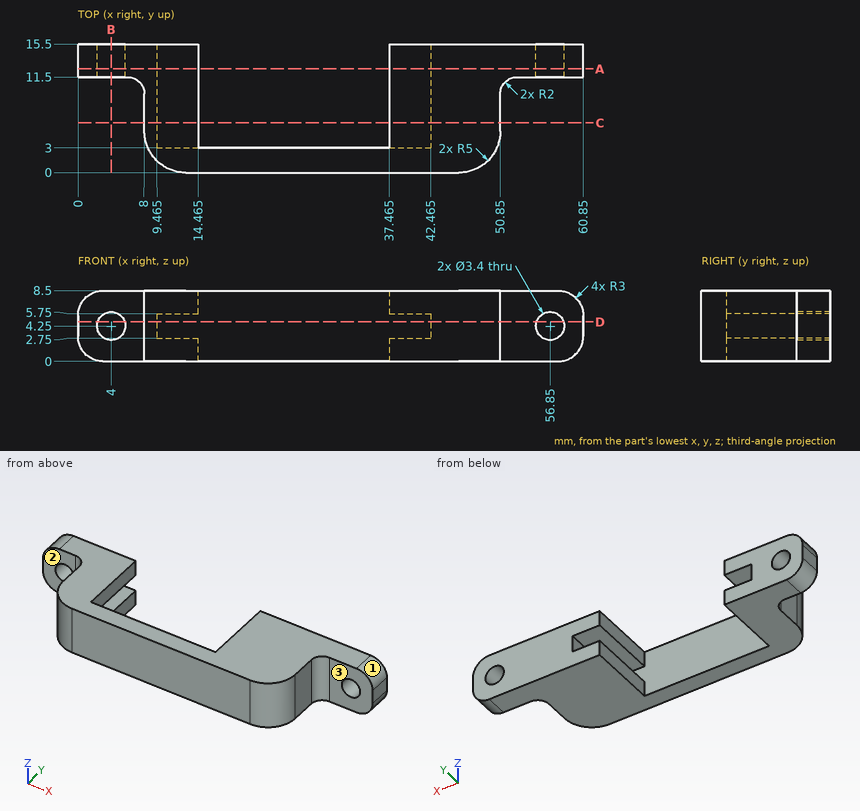
Part print with two shaded views. Sizes in mm from the minimum x, y, z corner. A direction names the side the tool comes from. Round coordinates to 2 decimals unless told otherwise and drop trailing zeros. Write each loop counter-clockwise with the first axis right and the second up, starting at its lowest first coordinate (ties: lowest second). Pieces come first, ordered by that corner, then holes. Notation, with made-up numbers: (41, -4) - (60, -4) arc R24 ccw to (60, 10) - close; hole circle Ø9 at (42.25, 81.5). An arc over 180 degrees is marked (long way). Use CSV: the item, a comma, the result in double quotes.
Item 1: Slice it at A-A, the plane y = 12.5. Write the cut outline in (x, z) (3 decimals), then the cut area to 3 significant figures.
Results list:
outline,"(0, 3) arc R3 ccw to (3, 0) - (14.465, 0) - (14.465, 2.75) - (9.465, 2.75) - (9.465, 5.75) - (14.465, 5.75) - (14.465, 8.5) - (3, 8.5) arc R3 ccw to (0, 5.5) - close; (37.465, 0) - (57.85, 0) arc R3 ccw to (60.85, 3) - (60.85, 5.5) arc R3 ccw to (57.85, 8.5) - (37.465, 8.5) - (37.465, 5.75) - (42.465, 5.75) - (42.465, 2.75) - (37.465, 2.75) - close; hole circle Ø3.4 at (4, 4.25); hole circle Ø3.4 at (56.85, 4.25)"
area,"266 mm²"
Item 2: Slice it at B-B, the plane x = 4. Write the cut outline in (y, z), then the cut area to 3 significant figures.
Results list:
outline,"(11.5, 0) - (15.5, 0) - (15.5, 2.55) - (11.5, 2.55) - close; (11.5, 5.95) - (15.5, 5.95) - (15.5, 8.5) - (11.5, 8.5) - close"
area,"20.4 mm²"
Item 3: Slice it at C-C, the plane y = 6. Write the cut outline in (x, z) (3 decimals), then the cut area to 3 significant figures.
Results list:
outline,"(8, 0) - (14.465, 0) - (14.465, 2.75) - (9.465, 2.75) - (9.465, 5.75) - (14.465, 5.75) - (14.465, 8.5) - (8, 8.5) - close; (37.465, 0) - (50.85, 0) - (50.85, 8.5) - (37.465, 8.5) - (37.465, 5.75) - (42.465, 5.75) - (42.465, 2.75) - (37.465, 2.75) - close"
area,"139 mm²"
Item 4: Tool access for the marked faces 1, 2 and 3: list every direction of +Z, -Z, +X, -X, +Y, -Y with a clear straight run to the whole face (end or side of a thin tool).
Results list:
face 1,"+Z, +X, +Y, -Y"
face 2,"+Z, -Z, -X, -Y"
face 3,"+Z, -Z, +X, -Y"
Item 5: Wall check: L1, parallel to X at y = 14, z = 4.25 (3 decimals); L2, parallel to X at y = 8.25, z = 6.75 (3 decimals); L3, parallel to Y at x = 13, z = 4.25. Give the ranges that are in metal, low to high.
Results list:
L1,"x = 0 to 2.3, 5.7 to 9.465, 42.465 to 55.15, 58.55 to 60.85"
L2,"x = 8 to 14.465, 37.465 to 50.85"
L3,"y = 0 to 3"
Item 6: Flat gauge pins, fed straight in: P1, Ø1.5, axis at y = 14, z = 1.5, coming from the +X side; P2, Ø1, axis at y = 5, z = 2.5, coming from the -X side; P3, Ø0.8, axis at y = 11.5, z = 7, coming from the +X side; P4, Ø2, axis at x = 4, z = 4.25, coming from the +Y side. Where does each tip first touch, or does it go through?
Results list:
P1,"stops at x = 60.75"
P2,"stops at x = 8"
P3,"stops at x = 60.64"
P4,"passes through"
Item 7: Slice it at D-D, the plane z = 4.75. Write the cut outline in (x, y) (3 decimals).
Results list:
outline,"(0, 11.5) - (2.375, 11.5) - (2.375, 15.5) - (0, 15.5) - close; (5.625, 11.5) - (6, 11.5) arc R2 cw to (8, 9.5) - (8, 5) arc R5 ccw to (13, 0) - (45.85, 0) arc R5 ccw to (50.85, 5) - (50.85, 9.5) arc R2 cw to (52.85, 11.5) - (55.225, 11.5) - (55.225, 15.5) - (42.465, 15.5) - (42.465, 3) - (9.465, 3) - (9.465, 15.5) - (5.625, 15.5) - close; (58.475, 11.5) - (60.85, 11.5) - (60.85, 15.5) - (58.475, 15.5) - close"
